```python
from build123d import *

# Parameters (mm, degrees)
F1_DEPTH = 8
F2_DEPTH = 7.5
F3_R     = 3.5
F4_SIZE  = 1


with BuildPart() as f1:
    # F0 (on Top) → F1 (new body)
    with BuildSketch(Plane.XY):
        Polygon((4.5, -37), (4.5, -4.5), (37, -4.5), (37, 3), (-3, 3), (-3, -37), align=None)
        Polygon((34, -1.5), (1.5, -1.5), (1.5, -34), (0, -34), (0, -1.5), (0, 0), (1.5, 0), (34, 0), align=None, mode=Mode.SUBTRACT)
    extrude(amount=F1_DEPTH)

    # F0 (on Top) → F2 (join)
    with BuildSketch(Plane.XY):
        Polygon((4.5, -37), (4.5, -4.5), (37, -4.5), (37, 3), (-3, 3), (-3, -37), align=None)
        Polygon((34, -1.5), (1.5, -1.5), (1.5, -34), (0, -34), (0, -1.5), (0, 0), (1.5, 0), (34, 0), align=None, mode=Mode.SUBTRACT)
        Polygon((1.5, -34), (1.5, -1.5), (34, -1.5), (34, 0), (1.5, 0), (0, 0), (0, -1.5), (0, -34), align=None)
    extrude(amount=-F2_DEPTH)

    # F3
    f3_edges = [f1.edges().sort_by_distance(p)[0] for p in [
        (20.75, -4.5, -7.5),
        (4.5, -20.75, -7.5),
        (17, 3, -7.5),
        (-3, -17, -7.5),
        (4.5, -4.5, 0.25),
        (-3, 3, 0.25),
        (0.75, -37, -7.5),
        (37, -0.75, -7.5),
        (4.5, -37, 0.25),
        (-3, -37, 0.25),
        (37, -4.5, 0.25),
        (37, 3, 0.25),
        (1.5, -1.5, 4),
    ]]
    fillet(f3_edges, radius=F3_R)

    # F4
    f4_edges = [f1.edges().sort_by_distance(p)[0] for p in [
        (0, -17, 8),
        (2.525126, -2.525126, 8),
        (17, 0, 8),
        (0.75, -34, 8),
        (34, -0.75, 8),
    ]]
    chamfer(f4_edges, length=F4_SIZE)


solid = f1.part
```
Here's how the part is built. I have some questions about the finished solid (model axes, mm). A direction names the side the tool comes from. Coordinates: 2 decimals unless noted, no trailing zeros. Order: outer loops, then holes, each group sorted by start corner. A loop starts at its lowest first (then second) coordinate and runs counter-clockwise, first axis right, second up. Notation, with made-up numbers: (27, 41.5) - (83, 41.5) arc R18 ccw to (83, 75.5) - close; hole circle Ø2 at (-18.75, 19). An arc over 180 degrees is marked (long way). One line per question, with ' | ' between items. Start each with the question number.
1. Which directions (+Z, -Z, +X, -X, +Y, -Y) give clear straight access to the entire face, cutting with the end or side of a thin tool? Please do faces 1 (the flat face through (1, -34, 3)), 2 (the cylindrical face through (20.93, -3.5, -6.45)), 3 (the flat face through (21, -4.5, 2)).
2. If we mould it in two halves opening along Y, with no side actions, what happens to faces 4 (the cylindrical face through (36, -3.45, 2.08)), 5 (the flat face through (19.8, -2, 7.5)), 6 (the cylindrical face through (2.5, -2.55, 3.55)), 7 (the flat face through (8, -3, 8))? For each: released by +Y, released by -Y, zero draft, split by the parting line, or undercut.
3. I'm going to push flat-ended pins straight in: pin 1 Ø8 at (y, z) = (-16, -2) entering from +X; pin 2 Ø7.5 at (x, z) = (12, 2.5) entering from -Y. Where does each tip first touch, or does it pass through?
4. If we section it at C-C (x = 21.5): Write out the boundary of the cut face in (y, z), and give its area (3 significant figures).
5. If we section it at A-A (z = 4.75): Write out the boundary of the cut face in (x, y), and give its area (3 significant figures).
6. Please list where these lines run through material, in increasing order: line 1 along X through (y, z) = (-29, 0.5); line 2 along Y through (x, z) = (31.5, 2.5); line 3 along X through (y, z) = (-1, 5.75). Write a range as [from, to].
7. If we section it at B-B (y = -26.5): Write out the boundary of the cut face in (x, z), and give its area (3 significant figures).
Model answer:
1) face 1: +Z | face 2: -Z, +X, -Y | face 3: +Z, -Z, +X, -Y
2) face 4: released by -Y | face 5: undercut | face 6: undercut | face 7: zero draft
3) pin 1: stops at x = 4.5 | pin 2: stops at y = -4.5
4) outline: (-4.5, -4) arc R3.5 ccw to (-1, -7.5) - (-0.5, -7.5) arc R3.5 ccw to (3, -4) - (3, 8) - (1, 8) - (0, 7) - (0, 0) - (-1.5, 0) - (-1.5, 7) - (-2.5, 8) - (-4.5, 8) - close | area: 98.0 mm²
5) outline: (-3, -33.5) arc R3.5 ccw to (0.5, -37) - (1, -37) arc R3.5 ccw to (4.5, -33.5) - (4.5, -8) arc R3.5 cw to (8, -4.5) - (33.5, -4.5) arc R3.5 ccw to (37, -1) - (37, -0.5) arc R3.5 ccw to (33.5, 3) - (0.5, 3) arc R3.5 ccw to (-3, -0.5) - close; hole (0, -34) - (1.5, -34) - (1.5, -5) arc R3.5 cw to (5, -1.5) - (34, -1.5) - (34, 0) - (0, 0) - close | area: 431 mm²
6) line 1: x = [-3, 0], [1.5, 4.5] | line 2: y = [-4.5, -1.5], [0, 3] | line 3: x = [-3, 0], [34, 37]
7) outline: (-3, -4) arc R3.5 ccw to (0.5, -7.5) - (1, -7.5) arc R3.5 ccw to (4.5, -4) - (4.5, 8) - (2.5, 8) - (1.5, 7) - (1.5, 0) - (0, 0) - (0, 7) - (-1, 8) - (-3, 8) - close | area: 98.0 mm²
